CAD build for the part. Positions are in the model's coordinates, mm. Face numbers are marked on the shaded views. A direction names the side the tool comes from. Coordinates: 2 decimals unless noted, no trailing zeros. Loops run counter-clockwise (first coordinate to the right, second up) from the corner with the lowest first, then second, coordinate; pieces in that order, holes last. Notation, with made-up numbers: M 32,64.5 L 61,64.5 A26 cw 61,92.5 Z; hole C 20.25,-2.75 d9. An arc over 180 degrees is marked long. Answer as a JSON object with one key per item and string values. Group by question number.
```python
from build123d import *

# Parameters (mm, degrees)
SKETCH1_R            = 2.1
BOSS_EXTRUDE1_DEPTH  = 65
SKETCH84_W           = 0.2
SKETCH84_H           = 5.6
BOSS_EXTRUDE8_DEPTH  = 40
SKETCH86_W           = 21.745720746
SKETCH86_H           = 21.517119214
CUT_EXTRUDE59_DEPTH  = 67.55103305
SKETCH87_W           = 20
SKETCH87_H           = 51.5
SKETCH87_W_2         = 10
SKETCH87_H_2         = 41.5
BOSS_EXTRUDE9_DEPTH  = 70
SKETCH88_W           = 17
SKETCH88_H           = 15
CUT_EXTRUDE60_DEPTH  = 5
SKETCH89_W           = 20
SKETCH89_H           = 51.5
BOSS_EXTRUDE10_DEPTH = 50
SKETCH90_W           = 10
SKETCH90_H           = 41.5
BOSS_EXTRUDE11_DEPTH = 5
SKETCH91_W           = 16
SKETCH91_H           = 47.5
CUT_EXTRUDE61_DEPTH  = 30
SKETCH92_W           = 70
SKETCH92_H           = 51.5
BOSS_EXTRUDE12_DEPTH = 40
BOSS_EXTRUDE13_DEPTH = 40
SKETCH94_W           = 13.084115127
SKETCH94_H           = 30.286066168
CUT_EXTRUDE62_DEPTH  = 40
SKETCH95_W           = 56
SKETCH95_H           = 47.5
CUT_EXTRUDE63_DEPTH  = 45
SKETCH97_W           = 37
SKETCH97_H           = 45.5
CUT_EXTRUDE64_DEPTH  = 45
SKETCH98_W           = 38
SKETCH98_H           = 47.5
CUT_EXTRUDE65_DEPTH  = 45


with BuildPart() as part:
    # Sketch1 → Boss-Extrude1 (new body)
    with BuildSketch(Plane(origin=(0, 0, 0), x_dir=(0, 0, -1), z_dir=(1, 0, 0))):
        with BuildLine():
            Line((-10, 9), (-10, 3))
            Line((-10, 3), (-8, 3))
            Line((-8, 3), (-8, 6))
            Line((-8, 6), (-7.060660172, 6))
            Line((-7.060660172, 6), (-4, 2.939339828))
            Line((-4, 2.939339828), (-4, -2.939339828))
            Line((-4, -2.939339828), (-7.060660172, -6))
            Line((-7.060660172, -6), (-8, -6))
            Line((-8, -6), (-8, -3))
            Line((-8, -3), (-10, -3))
            Line((-10, -3), (-10, -9))
            ThreePointArc((-10, -9), (-9.707106781, -9.707106781), (-9, -10))
            Line((-9, -10), (-3, -10))
            Line((-3, -10), (-3, -8))
            Line((-3, -8), (-6, -8))
            Line((-6, -8), (-6, -7.060660172))
            Line((-6, -7.060660172), (-2.939339828, -4))
            Line((-2.939339828, -4), (2.939339828, -4))
            Line((2.939339828, -4), (6, -7.060660172))
            Line((6, -7.060660172), (6, -8))
            Line((6, -8), (3, -8))
            Line((3, -8), (3, -10))
            Line((3, -10), (9, -10))
            ThreePointArc((9, -10), (9.707106781, -9.707106781), (10, -9))
            Line((10, -9), (10, -3))
            Line((10, -3), (8, -3))
            Line((8, -3), (8, -6))
            Line((8, -6), (7.060660172, -6))
            Line((7.060660172, -6), (4, -2.939339828))
            Line((4, -2.939339828), (4, 2.939339828))
            Line((4, 2.939339828), (7.060660172, 6))
            Line((7.060660172, 6), (8, 6))
            Line((8, 6), (8, 3))
            Line((8, 3), (10, 3))
            Line((10, 3), (10, 9))
            ThreePointArc((10, 9), (9.707106781, 9.707106781), (9, 10))
            Line((9, 10), (3, 10))
            Line((3, 10), (3, 8))
            Line((3, 8), (6, 8))
            Line((6, 8), (6, 7.060660172))
            Line((6, 7.060660172), (2.939339828, 4))
            Line((2.939339828, 4), (-2.939339828, 4))
            Line((-2.939339828, 4), (-6, 7.060660172))
            Line((-6, 7.060660172), (-6, 8))
            Line((-6, 8), (-3, 8))
            Line((-3, 8), (-3, 10))
            Line((-3, 10), (-9, 10))
            ThreePointArc((-9, 10), (-9.707106781, 9.707106781), (-10, 9))
        make_face()
        Circle(SKETCH1_R, mode=Mode.SUBTRACT)
    extrude(amount=BOSS_EXTRUDE1_DEPTH)

    # Sketch86 → Cut-Extrude59 (cut, through all)
    with BuildSketch(Plane(origin=(65, 0, 0), x_dir=(0, 0, -1), z_dir=(1, 0, 0))):
        with Locations((0.085738745, -0.242889128)):
            Rectangle(SKETCH86_W, SKETCH86_H)
    extrude(amount=-CUT_EXTRUDE59_DEPTH, mode=Mode.SUBTRACT)


with BuildPart() as body_2:
    # Sketch84 → Boss-Extrude8 (new body)
    with BuildSketch(Plane(origin=(65, 0, 0), x_dir=(0, 0, -1), z_dir=(1, 0, 0))):
        with Locations((-10.1, 0)):
            Rectangle(SKETCH84_W, SKETCH84_H)
        with Locations((-9.9, 0)):
            Rectangle(SKETCH84_W, SKETCH84_H)
        Polygon((-7.8, 5.8), (-7.143502884, 5.8), (-4.2, 2.856497116), (-4.2, -2.856497116), (-7.143502884, -5.8), (-7.8, -5.8), (-7.8, -2.8), (-9.8, -2.8), (-9.8, 2.8), (-7.8, 2.8), align=None)
    extrude(amount=BOSS_EXTRUDE8_DEPTH)

    # Sketch87 → Boss-Extrude9 (add)
    with BuildSketch(Plane.ZY.offset(-65)):
        with Locations((20.2, 12.95)):
            Rectangle(SKETCH87_W, SKETCH87_H)
        with Locations((20.2, 12.95)):
            Rectangle(SKETCH87_W_2, SKETCH87_H_2, mode=Mode.SUBTRACT)
    extrude(amount=-BOSS_EXTRUDE9_DEPTH)

    # Sketch88 → Cut-Extrude60 (cut)
    with BuildSketch(Plane(origin=(0, 38.7, 0), x_dir=(1, 0, 0), z_dir=(0, 1, 0))):
        with Locations((75.5, -20.2)):
            Rectangle(SKETCH88_W, SKETCH88_H)
    extrude(amount=-CUT_EXTRUDE60_DEPTH, mode=Mode.SUBTRACT)

    # Sketch89 → Boss-Extrude10 (add)
    with BuildSketch(Plane(origin=(135, 0, 0), x_dir=(0, 0, -1), z_dir=(1, 0, 0))):
        with Locations((-20.2, 12.95)):
            Rectangle(SKETCH89_W, SKETCH89_H)
    extrude(amount=-BOSS_EXTRUDE10_DEPTH)

    # Sketch90 → Boss-Extrude11 (add)
    with BuildSketch(Plane.ZY.offset(-85)):
        with Locations((20.2, 12.95)):
            Rectangle(SKETCH90_W, SKETCH90_H)
    extrude(amount=BOSS_EXTRUDE11_DEPTH)

    # Sketch91 → Cut-Extrude61 (cut)
    with BuildSketch(Plane(origin=(135, 0, 0), x_dir=(0, 0, -1), z_dir=(1, 0, 0))):
        with Locations((-20.2, 12.95)):
            Rectangle(SKETCH91_W, SKETCH91_H)
    extrude(amount=-CUT_EXTRUDE61_DEPTH, mode=Mode.SUBTRACT)

    # Sketch92 → Boss-Extrude12 (add)
    with BuildSketch(Plane.XY.offset(30.2)):
        with Locations((100, 12.95)):
            Rectangle(SKETCH92_W, SKETCH92_H)
    extrude(amount=BOSS_EXTRUDE12_DEPTH)

    # Sketch93 → Boss-Extrude13 (add)
    with BuildSketch(Plane.ZY.offset(-65)):
        Polygon((72.6, 2.8), (70.2, 2.8), (70.2, -2.8), (72.6, -2.8), (72.6, -5.8), (73.256497116, -5.8), (76.2, -2.856497116), (76.2, 2.856497116), (73.256497116, 5.8), (72.6, 5.8), align=None)
    extrude(amount=-BOSS_EXTRUDE13_DEPTH)

    # Sketch94 → Cut-Extrude62 (cut)
    with BuildSketch(Plane.ZY.offset(-65)):
        with Locations((3.657942437, 5.120137749)):
            Rectangle(SKETCH94_W, SKETCH94_H)
    extrude(amount=-CUT_EXTRUDE62_DEPTH, mode=Mode.SUBTRACT)

    # Sketch95 → Cut-Extrude63 (cut)
    with BuildSketch(Plane(origin=(135, 0, 0), x_dir=(0, 0, -1), z_dir=(1, 0, 0))):
        with Locations((-40.2, 12.95)):
            Rectangle(SKETCH95_W, SKETCH95_H)
    extrude(amount=-CUT_EXTRUDE63_DEPTH, mode=Mode.SUBTRACT)

    # Sketch97 → Cut-Extrude64 (cut)
    with BuildSketch(Plane.ZY.offset(-65)):
        with Locations((48.7, 12.95)):
            Rectangle(SKETCH97_W, SKETCH97_H)
    extrude(amount=-CUT_EXTRUDE64_DEPTH, mode=Mode.SUBTRACT)

    # Sketch98 → Cut-Extrude65 (cut)
    with BuildSketch(Plane(origin=(90, 0, 0), x_dir=(0, 0, -1), z_dir=(1, 0, 0))):
        with Locations((-49.2, 12.95)):
            Rectangle(SKETCH98_W, SKETCH98_H)
    extrude(amount=-CUT_EXTRUDE65_DEPTH, mode=Mode.SUBTRACT)


solid = body_2.part
```
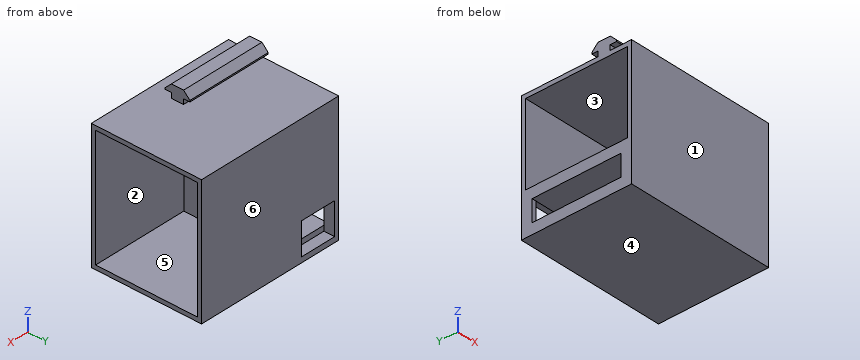
Item 1: Slice it at D-D, the plane x = 100.5. Write the cut outline in (y, z).
Item 2: Pull direction Z, two halves, no side cores. Call the marked faces 1, 2, 3 and 4: released by +Z, released by -Z, zero draft, split by the parting line, or undercut.
Item 3: Slice it at A-A, the plane x = 130.5. Write the cut outline in (y, z), then the cut area to 3 significant figures.
Item 4: Slice it at B-B, the plane y = 23. Write the cut outline in (x, z).
Item 5: Slice it at C-C, the plane z = 60. Write the cut outline in (x, y), then the cut area to 3 significant figures.
Item 6: Tool access for the marked faces 5 and 6: list every direction of +Z, -Z, +X, -X, +Y, -Y with a clear straight run to the whole face (end or side of a thin tool).
Item 7: Pin check, flat tips, straight feed: pin 1 (13.5 mm diameter, centred on x = 109, y = 16, fed in from +Z); pin 2 (5 mm diameter, centred on x = 74.5, z = 19, fed in from +Y); pin 3 (7.5 mm diameter, centred on x = 72, z = 18, fed in from +Y). Stop position of each tip, or through.
Item 8: Drill centre lines: L1, parallel to Z at x = 74.5, y = -6.5; L2, parallel to Y at x = 101.5, z = 62.5; L3, parallel to Z at x = 90.5, y = 25.5. Where is each one in solid material? Low to high. Write a range as from..to.
Computed:
{
 "1": {"outline": "M -12.8,10.2 L 38.7,10.2 L 38.7,70.2 L 2.8,70.2 L 2.8,72.6 L 5.8,72.6 L 5.8,73.26 L 2.86,76.2 L -2.86,76.2 L -5.8,73.26 L -5.8,72.6 L -2.8,72.6 L -2.8,70.2 L -12.8,70.2 Z; hole M -10.8,12.2 L 36.7,12.2 L 36.7,68.2 L -10.8,68.2 Z"},
 "2": {"face 1": "zero draft", "face 2": "undercut", "face 3": "undercut", "face 4": "released by -Z"},
 "3": {"outline": "M -12.8,10.2 L 38.7,10.2 L 38.7,70.2 L -12.8,70.2 Z; hole M -10.8,12.2 L 36.7,12.2 L 36.7,68.2 L -10.8,68.2 Z", "area": "430 mm2"},
 "4": {"outline": "M 65,10.2 L 135,10.2 L 135,12.2 L 90,12.2 L 90,30.2 L 65,30.2 L 65,25.2 L 80,25.2 L 80,15.2 L 65,15.2 Z; M 65,68.2 L 135,68.2 L 135,70.2 L 65,70.2 Z"},
 "5": {"outline": "M 65,-12.8 L 135,-12.8 L 135,-10.8 L 65,-10.8 Z; M 65,36.7 L 135,36.7 L 135,38.7 L 65,38.7 Z", "area": "280 mm2"},
 "6": {"face 5": "+X", "face 6": "+Z, -Z, +X, -X, +Y"},
 "7": {"pin 1": "z = 70.2", "pin 2": "y = -7.8", "pin 3": "y = 33.7"},
 "8": {"L1": "10.2..15.2, 25.2..30.2, 68.2..70.2", "L2": "-12.8..-10.8, 36.7..38.7", "L3": "10.2..12.2, 68.2..70.2"}
}
